Geometry check sheet. Reference: the model listing, model coordinates, mm. Coordinates: 2 decimals unless noted, no trailing zeros. Write each loop counter-clockwise with the first axis right and the second up, starting at its lowest first coordinate (ties: lowest second). Pieces come first, ordered by that corner, then holes. Notation, with made-up numbers: (77, -16) - (106, -16) arc R27 cw to (106, 6) - close; hole circle Ø7 at (27, -15.75). An arc over 180 degrees is marked (long way). Answer as a JSON object with one key per item and string values. Group by question number.
from build123d import *

# Parameters (mm, degrees)
SKETCH1_W           = 140
SKETCH1_H           = 100
BOSS_EXTRUDE1_DEPTH = 6.35
SKETCH2_R           = 12.705
CUT_EXTRUDE1_DEPTH  = 10
SKETCH3_R           = 1.5875
CUT_EXTRUDE2_DEPTH  = 10
CHAMFER1_SIZE       = 1


with BuildPart() as part:
    # Sketch1 → Boss-Extrude1 (new body)
    with BuildSketch(Plane(origin=(0, 0, 0), x_dir=(1, 0, 0), z_dir=(0, 1, 0))):
        with Locations((70, 50)):
            Rectangle(SKETCH1_W, SKETCH1_H)
    extrude(amount=BOSS_EXTRUDE1_DEPTH)

    # Sketch2 → Cut-Extrude1 (cut)
    with BuildSketch(Plane(origin=(0, 6.35, 0), x_dir=(1, 0, 0), z_dir=(0, 1, 0))):
        with Locations(Location((70, 50, 0), (0, 0, 270))):
            Circle(SKETCH2_R)
    extrude(amount=-CUT_EXTRUDE1_DEPTH, mode=Mode.SUBTRACT)

    # Sketch3 → Cut-Extrude2 (cut)
    with BuildSketch(Plane(origin=(0, 6.35, 0), x_dir=(1, 0, 0), z_dir=(0, 1, 0))):
        with Locations(Location((8.85, 50, 0), (0, 0, 270))):
            Circle(SKETCH3_R)
        with Locations(Location((131.15, 50, 0), (0, 0, 270))):
            Circle(SKETCH3_R)
    extrude(amount=-CUT_EXTRUDE2_DEPTH, mode=Mode.SUBTRACT)

    # Chamfer1
    chamfer1_edges = [part.edges().sort_by_distance(p)[0] for p in [
        (70, 6.35, -62.705),
    ]]
    chamfer(chamfer1_edges, length=CHAMFER1_SIZE)


solid = part.part
(1) Section check B-B (z = -50). Count the separate pieces of the cut face and the enclosed holes in it, and give its area (3 significant figures).
(2) Section check A-A (x = 131.15). Record the cut outline in (y, z).
(3) Material ranges on L1, parallel to X at y = 2.35, z = -50 (1 decimal); L2, parallel to Z at x = 131.15, y = 1.75; L3, parallel to Z at x = 69.5, y = 3.5, recorded low to high. Write a range as [from, to].
(4) Draft check along Z on faces 1 (the face through (129.74, 3.22, -49.27)), 2 (the face through (53, 0, -51)), 3 (the face through (69, 3, 0)), 4 (the face through (9.327, 3.219, -48.486)). Enter one of: +Z half, -Z half, draft (parallel to the pull), parting line (faces both ways), or undercut.
(5) Gauge pin test, flat end, axial feed: pin 1 (3.5 mm diameter, centred on x = 8.85, z = -50, fed in from +Y). Record the tip position at first contact, or that the pin passes through.
(6) Section check D-D (x = 70). Record the cut outline in (y, z) (3 decimals).
Conclusion:
{
 "1": {"separate pieces": "4", "enclosed holes": "0", "area": "686 mm^2"},
 "2": {"outline": "(0, -100) - (6.35, -100) - (6.35, -51.59) - (0, -51.59) - close; (0, -48.41) - (6.35, -48.41) - (6.35, 0) - (0, 0) - close"},
 "3": {"L1": "x = [0, 7.3], [10.4, 57.3], [82.7, 129.6], [132.7, 140]", "L2": "z = [-100, -51.59], [-48.41, 0]", "L3": "z = [-100, -62.7], [-37.3, 0]"},
 "4": {"face 1": "undercut", "face 2": "draft", "face 3": "+Z half", "face 4": "undercut"},
 "5": {"pin 1": "stops at y = 6.35"},
 "6": {"outline": "(0, -100) - (6.35, -100) - (6.35, -63.705) - (5.35, -62.705) - (0, -62.705) - close; (0, -37.295) - (5.35, -37.295) - (6.35, -36.295) - (6.35, 0) - (0, 0) - close"}
}
